Build history of the part. All positions in model axes, mm. A direction names the side the tool comes from. Round coordinates to 2 decimals unless told otherwise and drop trailing zeros. Write each loop counter-clockwise with the first axis right and the second up, starting at its lowest first coordinate (ties: lowest second). Pieces come first, ordered by that corner, then holes. Notation, with made-up numbers: (-19.75, 84.25) - (25.25, 84.25) arc R19 ccw to (25.25, 92.25) - close; hole circle Ø4 at (60, -4.5). An arc over 180 degrees is marked (long way). Write each question's results on one line, items separated by ' | '.
from build123d import *

# Parameters (mm, degrees)
F1_DEPTH = 19.05
F2_DEPTH = 19.05


with BuildPart() as f1:
    # F0 (on Right) → F1 (new body)
    with BuildSketch(Plane.YZ):
        Polygon((113.946683, 45.527574), (-38.453317, 45.527574), (-140.053317, -411.672426), (-140.053317, -430.722426), (-89.253317, -430.722426), (-89.253317, -411.672426), (-38.453317, -411.672426), (-38.453317, -430.722426), (12.346683, -430.722426), (12.346683, -411.672426), (63.146683, -411.672426), (63.146683, -430.722426), (113.946683, -430.722426), (113.946683, -411.672426), (113.946683, -335.472426), (113.946683, -259.272426), (113.946683, -183.072426), (113.946683, -106.872426), (113.946683, -30.672426), align=None)
        Polygon((22.834336, -239.086572), (41.703042, -241.708486), (31.215389, -317.18331), (12.346683, -314.561397), align=None, mode=Mode.SUBTRACT)
        Polygon((43.809643, -88.136923), (62.678349, -90.758837), (52.190696, -166.233661), (33.32199, -163.611748), align=None, mode=Mode.SUBTRACT)
    extrude(amount=F1_DEPTH)

    # F0 (on Right) → F2 (join)
    with BuildSketch(Plane.YZ):
        Polygon((113.946683, 45.527574), (-38.453317, 45.527574), (-140.053317, -411.672426), (-140.053317, -430.722426), (-89.253317, -430.722426), (-89.253317, -411.672426), (-38.453317, -411.672426), (-38.453317, -430.722426), (12.346683, -430.722426), (12.346683, -411.672426), (63.146683, -411.672426), (63.146683, -430.722426), (113.946683, -430.722426), (113.946683, -411.672426), (113.946683, -335.472426), (113.946683, -259.272426), (113.946683, -183.072426), (113.946683, -106.872426), (113.946683, -30.672426), align=None)
        Polygon((22.834336, -239.086572), (41.703042, -241.708486), (31.215389, -317.18331), (12.346683, -314.561397), align=None, mode=Mode.SUBTRACT)
        Polygon((43.809643, -88.136923), (62.678349, -90.758837), (52.190696, -166.233661), (33.32199, -163.611748), align=None, mode=Mode.SUBTRACT)
    extrude(amount=F2_DEPTH)


solid = f1.part
(1) Slice it at D-D, the plane y = -100.5. Write the cut outline in (x, z), and give its area (3 significant figures).
Worked answers:
outline: (0, -430.72) - (19.05, -430.72) - (19.05, -233.68) - (0, -233.68) - close | area: 3,750 mm2
(2) Flat gauge pins, fed straight in: pin 1 Ø10 at (x, z) = (12, -184.5) entering from -Y; pin 2 Ø10 at (x, z) = (16, -104) entering from -Y; pin 3 Ø5.5 at (x, y) = (9, -56) entering from -Z. Where does each tip first touch, or does it go through?
Worked answers:
pin 1: stops at y = -90.68 | pin 2: stops at y = -72.79 | pin 3: stops at z = -411.67
(3) Slice it at A-A, the plane x = 3.75. Write the cut outline in (y, z), and give its area (3 significant figures).
Worked answers:
outline: (-140.05, -430.72) - (-89.25, -430.72) - (-89.25, -411.67) - (-38.45, -411.67) - (-38.45, -430.72) - (12.35, -430.72) - (12.35, -411.67) - (63.15, -411.67) - (63.15, -430.72) - (113.95, -430.72) - (113.95, 45.53) - (-38.45, 45.53) - (-140.05, -411.67) - close; hole (12.35, -314.56) - (31.22, -317.18) - (41.7, -241.71) - (22.83, -239.09) - close; hole (33.32, -163.61) - (52.19, -166.23) - (62.68, -90.76) - (43.81, -88.14) - close | area: 92,900 mm2
(4) Drill centre lines: probe 1 along Z at (x, y) = (14.75, 23); probe 2 along Y at (x, z) = (1.5, -121); probe 3 along Y at (x, z) = (10.75, -308.5). Where is each one in solid material? Low to high. Write a range as [from, to].
Worked answers:
probe 1: z = [-411.67, -316.04], [-239.11, 45.53] | probe 2: y = [-75.46, 39.24], [58.48, 113.95] | probe 3: y = [-117.13, 13.19], [32.42, 113.95]
(5) Slice it at B-B, the plane z = -148. Write the cut outline in (x, y).
Worked answers:
outline: (0, -81.46) - (19.05, -81.46) - (19.05, 35.49) - (0, 35.49) - close; (0, 54.72) - (19.05, 54.72) - (19.05, 113.95) - (0, 113.95) - close
(6) Tool access for faces 5 (the flat face through (9, -89.253, -421)), 6 (the flat face through (9.392, 36.533, -278.918)), 7 (the flat face through (9, -115, -430.722)): list every direction of +Z, -Z, +X, -X, +Y, -Y with a clear straight run to the whole face (end or side of a thin tool).
Worked answers:
face 5: -Z, +X, -X | face 6: +X, -X | face 7: -Z, +X, -X, +Y, -Y
(7) Two-plate mould, pull along Z, no slides. Class faces 1 (the flat face through (9, 113.947, -196)), 2 (the flat face through (9.39, 53.11, -89.43)), 3 (the flat face through (9, 39, 45.528)), 4 (the flat face through (9.39, 21.91, -315.89)): released by +Z, released by -Z, zero draft, split by the parting line, or undercut.
Worked answers:
face 1: zero draft | face 2: undercut | face 3: released by +Z | face 4: undercut
(8) Slice it at C-C, the plane z = -289.5. Write the cut outline in (x, y).
Worked answers:
outline: (0, -112.9) - (19.05, -112.9) - (19.05, 15.83) - (0, 15.83) - close; (0, 35.06) - (19.05, 35.06) - (19.05, 113.95) - (0, 113.95) - close
